For this review, take the finished solid that the model builds, in its own axes (mm). Give positions to 0.01 mm unless a question says otherwise; leave off trailing zeros. Loops run counter-clockwise (first coordinate to the right, second up) from the corner with the lowest first, then second, coordinate; pieces in that order, holes last.
```python
from build123d import *

# Parameters (mm, degrees)
SKETCH_2_R          = 100
EXTRUDE_1_DEPTH     = 40
CUT_EXTRUDE_1_DEPTH = 30
SKETCH_4_R          = 3
EXTRUDE_2_DEPTH     = 74


with BuildPart() as part:
    # 草图2 → 凸台-拉伸1 (new body)
    with BuildSketch(Plane.XY):
        Circle(SKETCH_2_R)
    extrude(amount=EXTRUDE_1_DEPTH)

    # 草图3 → 切除-拉伸1 (cut)
    with BuildSketch(Plane.XY.offset(40)):
        Polygon((0, -100), (35, -100), (35, 100), (-35, 100), (-35, -100), align=None)
    extrude(amount=-CUT_EXTRUDE_1_DEPTH, mode=Mode.SUBTRACT)

    # 草图4 → 凸台-拉伸2 (add)
    with BuildSketch(Plane(origin=(-35, 0, 0), x_dir=(0, 0, -1), z_dir=(1, 0, 0))):
        with Locations(Location((-25, 78.674969976, 0), (0, 0, 180))):
            Circle(SKETCH_4_R)
    extrude(amount=EXTRUDE_2_DEPTH)


solid = part.part
```
Item 1: Take a section at A-A on z = 25. Give the boundary of the cut face in (x, y).
Answer:
outline: (-35, -93.67) - (-35, 75.67) - (35, 75.67) - (35, -93.67) arc R100 ccw to (35, 93.67) - (35, 81.67) - (-35, 81.67) - (-35, 93.67) arc R100 ccw to start
Item 2: Take a section at D-D on y = 0. Give the boundary of the cut face in (x, z).
Answer:
outline: (-100, 0) - (100, 0) - (100, 40) - (35, 40) - (35, 10) - (-35, 10) - (-35, 40) - (-100, 40) - close
Item 3: Take a section at C-C on z = 13. Give the boundary of the cut face in (x, y), and give its area (3 significant figures).
Answer:
outline: (-35, -93.67) - (-35, 93.67) arc R100 ccw to start; (35, -93.67) arc R100 ccw to (35, 93.67) - close
area: 17,700 mm2
Item 4: Clearance check with flat-ended pins moving along their axes: pin 1 Ø2 at (y, z) = (15, 17) entering from +X; pin 2 Ø9 at (y, z) = (39, 31.5) entering from -X; pin 3 Ø9 at (y, z) = (3, 21) entering from +X; pin 4 Ø4 at (x, z) = (-53, 32.5) entering from -Y. State where each tip first meets the part, or that it passes through.
Answer:
pin 1: stops at x = 99.02
pin 2: stops at x = -93.86
pin 3: stops at x = 100
pin 4: stops at y = -86.02
Item 5: The part is to be moulded in two halves that separate along X. For faces 1 (the flat face through (-1, 1, 0)), 2 (the cylindrical face through (95.38, 30.04, 19.72)), 3 (the cylindrical face through (-0.49, 81.604, 24.35)), 4 (the flat face through (0, 1, 10)), say which applies: released by +X, released by -X, zero draft, split by the parting line, or undercut.
Answer:
face 1: zero draft
face 2: split by the parting line
face 3: undercut
face 4: undercut
Item 6: Take a section at B-B on x = -24.5. Give the boundary of the cut face in (y, z).
Answer:
outline: (-96.95, 0) - (96.95, 0) - (96.95, 10) - (-96.95, 10) - close; circle Ø6 at (78.67, 25)
Item 7: For L1, parallel to X at y = -33, z = 26; L2, parallel to X at y = -56.5, z = 16; L3, parallel to Z at x = -2, y = 89.5, list the stretches that pass through material, from the lowest coordinate up.
Answer:
L1: x = -94.4 to -35, 35 to 94.4
L2: x = -82.51 to -35, 35 to 82.51
L3: z = 0 to 10
